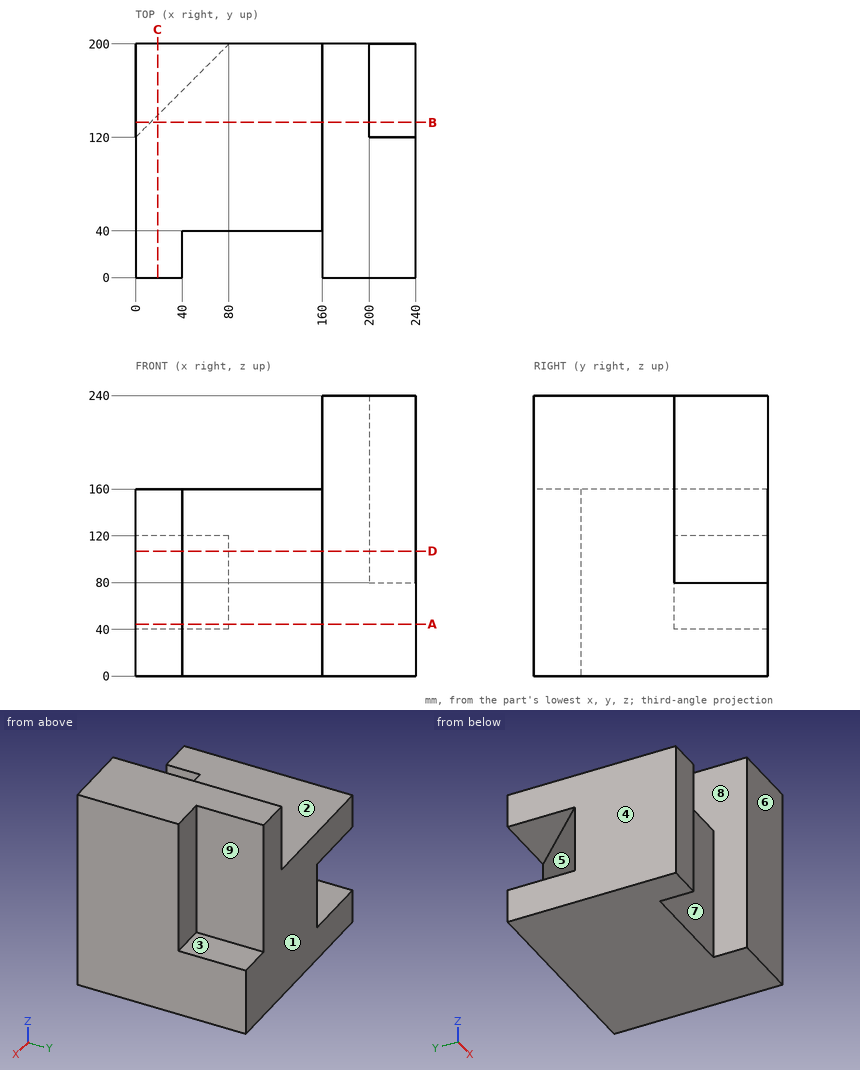
Verification items for this drawing (mm, ordinates from the low corner). A direction names the side the tool comes from. Give positions to 0.01 mm unless a question says otherwise; leave off trailing zeros. Order: outer loops, then holes, each group sorted by start corner. A loop starts at its lowest first (then second) coordinate and runs counter-clockwise, first axis right, second up. Notation, with made-up numbers: M 77,49 L 118,49 A13 ccw 118,72 Z; hole C 23,54.5 d6. An arc over 180 degrees is marked long. Use a Markdown table: item, result.
Item 1: Section check D-D (z = 107). Record the cut outline in (x, y).
Answers follow:
| item | result |
|---|---|
| outline | M 0,0 L 40,0 L 40,40 L 160,40 L 160,0 L 240,0 L 240,120 L 200,120 L 200,200 L 80,200 L 0,120 Z |
Item 2: Section check C-C (x = 19). Record the cut outline in (y, z).
Answers follow:
| item | result |
|---|---|
| outline | M 0,0 L 200,0 L 200,40 L 139,40 L 139,120 L 200,120 L 200,160 L 0,160 Z |
Item 3: Tool access check on the marked faces 1, 2, 3, 4 and 5. Record the directions out of +Z, -Z, +X, -X, +Y, -Y that give a thin tool (end or side, any length) a straight path to the whole face; none if there is none.
Answers follow:
| item | result |
|---|---|
| face 1 | +Z, -Z, +X, -X, +Y |
| face 2 | +Z, -X, +Y, -Y |
| face 3 | +Z, +X, +Y |
| face 4 | +Z, -Z, -X, +Y, -Y |
| face 5 | -X, +Y |
Item 4: Section check B-B (y = 133). Record the cut outline in (x, z), and give its area (3 significant figures).
Answers follow:
| item | result |
|---|---|
| outline | M 0,0 L 240,0 L 240,80 L 200,80 L 200,240 L 160,240 L 160,160 L 0,160 L 0,120 L 13,120 L 13,40 L 0,40 Z |
| area | 37,400 mm2 |
Item 5: Section check A-A (z = 44.5). Record the cut outline in (x, y).
Answers follow:
| item | result |
|---|---|
| outline | M 0,0 L 40,0 L 40,40 L 160,40 L 160,0 L 240,0 L 240,200 L 80,200 L 0,120 Z |
Item 6: Depth check by flat-ended pin: P1, Ø20, axis at x = 214, y = 177.5, coming from the +Z side; P2, Ø24, axis at x = 21, y = 164.5, coming from the +Z side. Enter the tip coordinate at first touch or a pass-through.
Answers follow:
| item | result |
|---|---|
| P1 | stops at z = 80 |
| P2 | stops at z = 160 |
Item 7: Material ranges on line 1 along X through (y, z) = (36.5, 124.5); line 2 along Z through (x, y) = (15, 50.5); line 3 along X through (y, z) = (164, 184.5), recorded low to high.
Answers follow:
| item | result |
|---|---|
| line 1 | x = 0 to 40, 160 to 240 |
| line 2 | z = 0 to 160 |
| line 3 | x = 160 to 200 |
Item 8: Draft check along X on the marked faces 6, 7, 8 and 9. Enter one of: +X half, -X half, draft (parallel to the pull), parting line (faces both ways), or undercut.
Answers follow:
| item | result |
|---|---|
| face 6 | draft |
| face 7 | undercut |
| face 8 | undercut |
| face 9 | +X half |
